Geometry check sheet. Reference: the model listing, model coordinates, mm. Round coordinates to 2 decimals unless told otherwise and drop trailing zeros. Loops run counter-clockwise (first coordinate to the right, second up) from the corner with the lowest first, then second, coordinate; pieces in that order, holes last. Notation, with made-up numbers: M -39,-22 L -3,-22 A27 cw -3,2 Z; hole C 86.5,61.25 d3. An arc over 180 degrees is marked long. Write item = value, one per line.
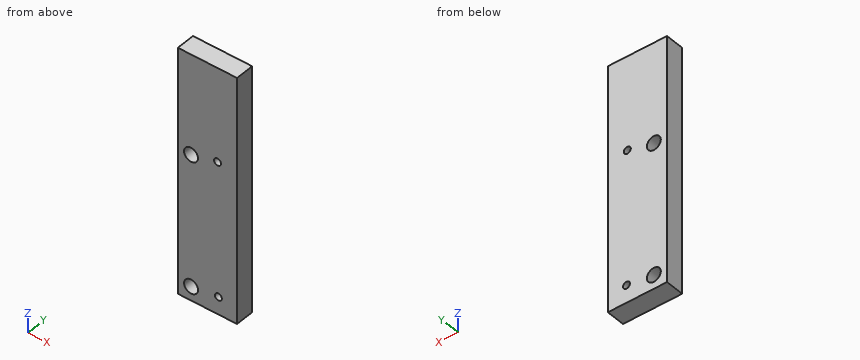
from build123d import *

# Parameters (mm, degrees)
F0_W     = 27.0002
F0_H     = 111.9886
F0_R     = 3.175
F0_R_2   = 1.5875
F1_DEPTH = 8.5


with BuildPart() as f1:
    # F0 (on Front) → F1 (new body)
    with BuildSketch(Plane.XZ):
        with Locations((-48.265494, -24.59839)):
            Rectangle(F0_W, F0_H)
        with Locations((-55.745794, -74.24269)):
            Circle(F0_R, mode=Mode.SUBTRACT)
        with Locations((-43.274394, -72.59169)):
            Circle(F0_R_2, mode=Mode.SUBTRACT)
        with Locations((-55.745794, -14.24789)):
            Circle(F0_R, mode=Mode.SUBTRACT)
        with Locations((-43.655394, -11.37769)):
            Circle(F0_R_2, mode=Mode.SUBTRACT)
    extrude(amount=-F1_DEPTH)


solid = f1.part
(1) Material ranges on line 1 along Z through (x, y) = (-55.5, 2.25); line 2 along Z through (x, y) = (-57, 1.75); line 3 along X through (y, z) = (4, -72), recorded low to high. Write a range as from..to.
Result set:
line_1 = -80.59..-77.41, -71.08..-17.41, -11.08..31.4
line_2 = -80.59..-77.16, -71.33..-17.16, -11.33..31.4
line_3 = -61.77..-57.99, -53.5..-44.75, -41.8..-34.77
(2) Sectioned sample at B-B on y = 1.75. State how many separate pieces and enclosed holes the cut face has, then the cut area to 3 significant figures.
Result set:
separate_pieces = 1
enclosed_holes = 4
area = 2,940 mm2
(3) Depth check by flat-ended pin: pin 1 Ø5 at (x, z) = (-43.27, -72.59) entering from -Y; pin 2 Ø2.5 at (x, z) = (-43.66, -11.38) entering from +Y. Enter the tip coordinate at first touch or a pass-through.
Result set:
pin_1 = 0
pin_2 = through
(4) Sectioned sample at A-A on x = -55.75. Record the cut outline in (y, z), then the cut area to 3 significant figures.
Result set:
outline = M 0,-80.59 L 8.5,-80.59 L 8.5,-77.42 L 0,-77.42 Z; M 0,-71.07 L 8.5,-71.07 L 8.5,-17.42 L 0,-17.42 Z; M 0,-11.07 L 8.5,-11.07 L 8.5,31.4 L 0,31.4 Z
area = 844 mm2
